Drawing for the job (mm, zero at the part's lowest x, y, z). Coordinates: 2 decimals unless noted, no trailing zeros. Write each loop counter-clockwise with the first axis right and the second up, starting at its lowest first coordinate (ties: lowest second). Pieces come first, ordered by that corner, then holes. Notation, with made-up numbers: M 13.5,69.5 L 55.5,69.5 A26 cw 55.5,87.5 Z; hole C 77.5,37 d4. An arc over 180 degrees is marked long. Use a Markdown table: item, result. Add a question column.
Q1. Slice it at D-D on z = 5.75. Write the cut outline in (x, y).
Q2. Mould opens along Z. For the marked faces 1, 2, 3 and 4 say: released by +Z, released by -Z, zero draft, split by the parting line, or undercut.
Q3. Slice it at B-B on x = 4.75. Write the cut outline in (y, z) (1 decimal).
Q4. Pin check, flat tips, straight feed: pin 1 Ø1 at (y, z) = (1, 7) entering from +X (1 decimal); pin 2 Ø1 at (y, z) = (0.5, 2.5) entering from +X (1 decimal). Stop position of each tip, or through.
Q5. Slice it at A-A on z = 4.75. Write the cut outline in (x, y) (1 decimal).
Q6. Slice it at C-C on y = 1.7. Write the cut outline in (x, z) (1 decimal).
Q7. Wall check: L1, parallel to Z at x = 4.5, y = 0.3 (1 decimal); L2, parallel to Z at x = 4, y = 2.1 (1 decimal); L3, parallel to X at y = 0.2, z = 3 (1 decimal). Give the ranges that are in metal, low to high. Write a range as from..to.
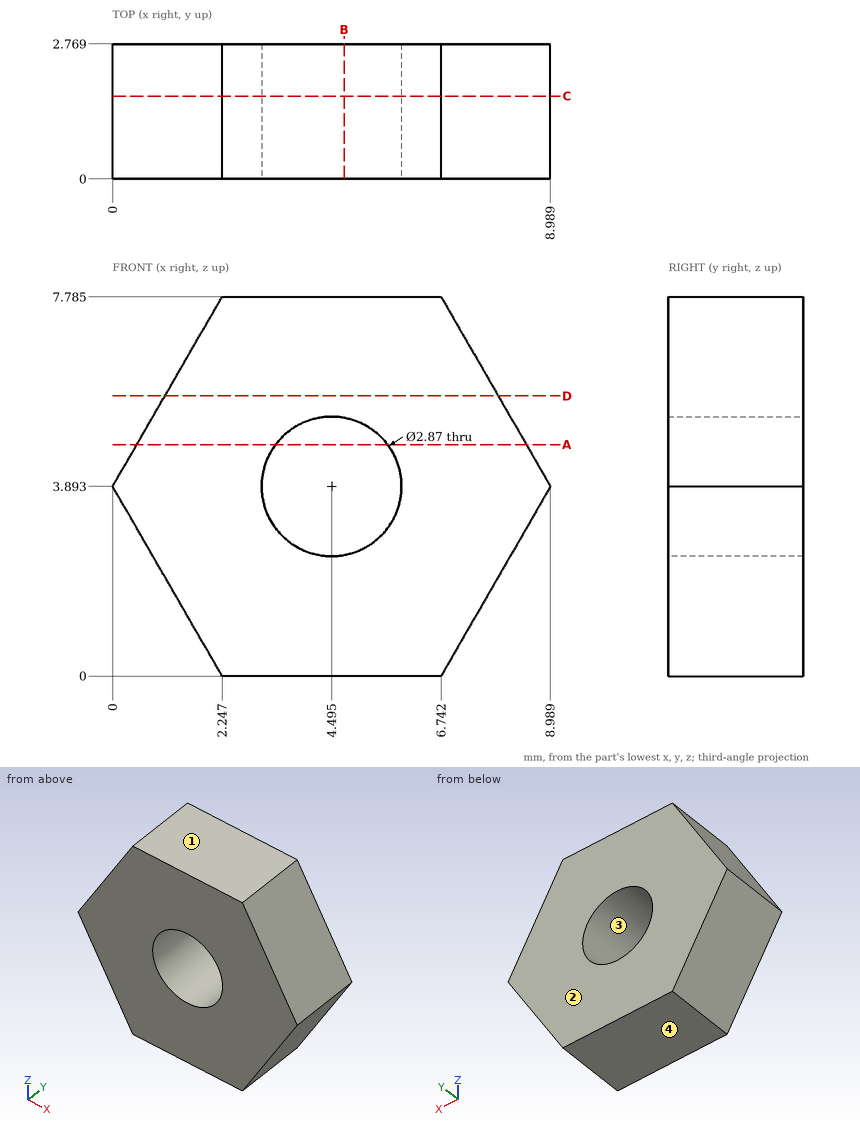
Recorded:
| question | item | result |
|---|---|---|
| 1 | outline | M 1.07,0 L 7.92,0 L 7.92,2.77 L 1.07,2.77 Z |
| 2 | face 1 | released by +Z |
| 2 | face 2 | zero draft |
| 2 | face 3 | undercut |
| 2 | face 4 | released by -Z |
| 3 | outline | M 0,0 L 2.8,0 L 2.8,2.5 L 0,2.5 Z; M 0,5.3 L 2.8,5.3 L 2.8,7.8 L 0,7.8 Z |
| 4 | pin 1 | x = 7.5 |
| 4 | pin 2 | x = 8.5 |
| 5 | outline | M 0.5,0 L 3.3,0 L 3.3,2.8 L 0.5,2.8 Z; M 5.6,0 L 8.5,0 L 8.5,2.8 L 5.6,2.8 Z |
| 6 | outline | M 0,3.9 L 2.2,0 L 6.7,0 L 9,3.9 L 6.7,7.8 L 2.2,7.8 Z; hole C 4.5,3.9 d2.9 |
| 7 | L1 | 0..2.5, 5.3..7.8 |
| 7 | L2 | 0..2.5, 5.2..7.8 |
| 7 | L3 | 0.5..3.4, 5.6..8.5 |
